```python
from build123d import *

# Parameters (mm, degrees)
SKETCH_1_W           = 20
SKETCH_1_H           = 12
SKETCH_1_R           = 1.65
EXTRUDE_1_DEPTH      = 4
SKETCH_2_W           = 20
SKETCH_2_H           = 3
EXTRUDE_2_DEPTH      = 84
EXTRUDE_3_DEPTH      = 1
EXTRUDE_3_DEPTH_BACK = 1
SKETCH_4_R           = 1.65
CUT_EXTRUDE_1_DEPTH  = 3


with BuildPart() as part:
    # 草图1 → 凸台-拉伸1 (new body)
    with BuildSketch(Plane(origin=(0, 0, 0), x_dir=(1, 0, 0), z_dir=(0, 1, 0))):
        Rectangle(SKETCH_1_W, SKETCH_1_H)
        with Locations(Location((-5.65, 0, 0), (0, 0, 270))):
            Circle(SKETCH_1_R, mode=Mode.SUBTRACT)
        with Locations(Location((5.65, 0, 0), (0, 0, 270))):
            Circle(SKETCH_1_R, mode=Mode.SUBTRACT)
    extrude(amount=EXTRUDE_1_DEPTH)

    # 草图2 → 凸台-拉伸2 (add)
    with BuildSketch(Plane(origin=(0, 0, 0), x_dir=(1, 0, 0), z_dir=(0, 1, 0))):
        with Locations((0, 7.5)):
            Rectangle(SKETCH_2_W, SKETCH_2_H)
    extrude(amount=EXTRUDE_2_DEPTH)

    # 草图3 → 凸台-拉伸3 (add, two sides: drawn at the far end of the back side and taken through both)
    with BuildSketch(Plane(origin=(0, 0, 0), x_dir=(0, 0, -1), z_dir=(1, 0, 0)).offset(-EXTRUDE_3_DEPTH_BACK)):
        Polygon((-2, 4), (6, 4), (6, 29), align=None)
    extrude(amount=EXTRUDE_3_DEPTH + EXTRUDE_3_DEPTH_BACK)

    # 草图4 → 切除-拉伸1 (cut)
    with BuildSketch(Plane.XY.offset(-6)):
        with Locations((0, 39)):
            Circle(SKETCH_4_R)
        with Locations((0, 49)):
            Circle(SKETCH_4_R)
        with Locations((0, 59)):
            Circle(SKETCH_4_R)
        with Locations((0, 69)):
            Circle(SKETCH_4_R)
        with Locations((0, 79)):
            Circle(SKETCH_4_R)
    extrude(amount=-CUT_EXTRUDE_1_DEPTH, mode=Mode.SUBTRACT)


solid = part.part
```
Geometry: final body of the model. Coordinates: model frame, mm. A direction names the side the tool comes from. Coordinates: 2 decimals unless noted, no trailing zeros. Order: outer loops, then holes, each group sorted by start corner. A loop starts at its lowest first (then second) coordinate and runs counter-clockwise, first axis right, second up. Notation, with made-up numbers: (48.25, 38.5) -> (53.25, 38.5) arc R18 cw to (53.25, 64.5) -> close; hole circle Ø11 at (-32.5, 82.25). An arc over 180 degrees is marked (long way). Answer in a Markdown table with one row per item.
Item 1: Draft query along X for faces 1 (the flat face through (1, 11, -4)), 2 (the flat face through (0, 84, -8)), 3 (the flat face through (-1, 11, -4)), 4 (the cylindrical face through (-0.4, 77.4, -7.5)). Return one class per face: released by +X, released by -X, zero draft, split by the parting line, or undercut.
Return value:
| item | result |
|---|---|
| face 1 | released by +X |
| face 2 | zero draft |
| face 3 | released by -X |
| face 4 | undercut |
Item 2: Section A-A on y = 69. Output: boundary loops of the cut face in (x, z), plus the area to 3 significant figures.
Return value:
| item | result |
|---|---|
| outline | (-10, -9) -> (-1.65, -9) -> (-1.65, -6) -> (-10, -6) -> close; (1.65, -9) -> (10, -9) -> (10, -6) -> (1.65, -6) -> close |
| area | 50.1 mm² |
Item 3: Contact query for flat-ended pins moving along their axis: P1, Ø6, axis at y = 24, z = -2.5, coming from the -X side; P2, Ø4, axis at x = -7, z = 1.5, coming from the +Y side; P3, Ø2.5, axis at x = 5.65, z = 0, coming from the +Y side; P4, Ø8, axis at x = -3.5, y = 53.5, coming from the +Z side. Output: stop coordinate, or through.
Return value:
| item | result |
|---|---|
| P1 | stops at x = -1 |
| P2 | stops at y = 4 |
| P3 | passes through |
| P4 | stops at z = -6 |
Item 4: Access query for faces 5 (the flat face through (-10, 36, -7)), 6 (the flat face through (-2, 4, 0)). Directions: +Z, -Z, +X, -X, +Y, -Y. A direction counts if a zero-diameter tool reaches every point of the face in a straight line with its end or side. Return the directions, or none.
Return value:
| item | result |
|---|---|
| face 5 | +Z, -Z, -X, +Y, -Y |
| face 6 | +Z, +Y |
Item 5: Section B-B on z = 0. Output: boundary loops of the cut face in (x, y), plus the area to 3 significant figures.
Return value:
| item | result |
|---|---|
| outline | (-10, 0) -> (-7.3, 0) -> (-7.3, 4) -> (-10, 4) -> close; (-4, 0) -> (4, 0) -> (4, 4) -> (1, 4) -> (1, 10.25) -> (-1, 10.25) -> (-1, 4) -> (-4, 4) -> close; (7.3, 0) -> (10, 0) -> (10, 4) -> (7.3, 4) -> close |
| area | 66.1 mm² |
Item 6: Section C-C on y = 16.5. Output: boundary loops of the cut face in (x, z).
Return value:
| item | result |
|---|---|
| outline | (-10, -9) -> (10, -9) -> (10, -6) -> (1, -6) -> (1, -2) -> (-1, -2) -> (-1, -6) -> (-10, -6) -> close |
Item 7: Ray query, L1, parallel to Y at x = 0, z = -8.05; L2, parallel to X at y = 0.8, z = 0; L3, parallel to X at y = 79, z = -7.65. Return the intervals inside material, ascending.
Return value:
| item | result |
|---|---|
| L1 | y = 0 to 37.35, 40.65 to 47.35, 50.65 to 57.35, 60.65 to 67.35, 70.65 to 77.35, 80.65 to 84 |
| L2 | x = -10 to -7.3, -4 to 4, 7.3 to 10 |
| L3 | x = -10 to -1.65, 1.65 to 10 |
Item 8: Section D-D on z = -4. Output: boundary loops of the cut face in (x, y), plus the area to 4 significant figures.
Return value:
| item | result |
|---|---|
| outline | (-10, 0) -> (10, 0) -> (10, 4) -> (1, 4) -> (1, 22.75) -> (-1, 22.75) -> (-1, 4) -> (-10, 4) -> close |
| area | 117.5 mm² |
